```python
from build123d import *

# Parameters (mm, degrees)
SKETCH1_W           = 400
SKETCH1_H           = 76.2
BOSS_EXTRUDE1_DEPTH = 50.8
SKETCH3_R           = 6.75
CUT_EXTRUDE2_DEPTH  = 50.8
SKETCH5_R           = 16
CUT_EXTRUDE3_DEPTH  = 77.2


with BuildPart() as part:
    # Sketch1 → Boss-Extrude1 (new body)
    with BuildSketch(Plane(origin=(0, 0, 0), x_dir=(1, 0, 0), z_dir=(0, 1, 0))):
        with Locations((200, 38.1)):
            Rectangle(SKETCH1_W, SKETCH1_H)
    extrude(amount=BOSS_EXTRUDE1_DEPTH)

    # Sketch3 → Cut-Extrude2 (cut)
    with BuildSketch(Plane(origin=(0, 50.8, 0), x_dir=(1, 0, 0), z_dir=(0, 1, 0))):
        with Locations((25, 63)):
            Circle(SKETCH3_R)
        with Locations((25, 13)):
            Circle(SKETCH3_R)
        with Locations((375, 63)):
            Circle(SKETCH3_R)
        with Locations((375, 13)):
            Circle(SKETCH3_R)
    extrude(amount=-CUT_EXTRUDE2_DEPTH, mode=Mode.SUBTRACT)

    # Sketch5 → Cut-Extrude3 (cut, through all)
    with BuildSketch(Plane.XY):
        with Locations((200, 30)):
            Circle(SKETCH5_R)
        with Locations((70, 30)):
            Circle(SKETCH5_R)
        with Locations((330, 30)):
            Circle(SKETCH5_R)
    extrude(amount=-CUT_EXTRUDE3_DEPTH, mode=Mode.SUBTRACT)


solid = part.part
```
For this review, take the finished solid that the model builds, in its own axes (mm). Give positions to 0.01 mm unless a question says otherwise; leave off trailing zeros. Write each loop counter-clockwise with the first axis right and the second up, starting at its lowest first coordinate (ties: lowest second). Pieces come first, ordered by that corner, then holes.
Item 1: Take a section at A-A (x = 375). Give the boundary of the cut face in (y, z), and give its area (3 significant figures).
Item 2: Take a section at B-B (z = -63). Give the boundary of the cut face in (x, y).
Item 3: Wall thickness on probe 1 along Z at (x, y) = (374, 24); probe 2 along X at (y, z) = (29.5, -20); probe 3 along X at (y, z) = (9, -18): over which ranges is each line inside the solid? List them lowest first.
Item 4: The part is to be moulded in two halves that separate along X. For faces 1 (the face through (0, 25, -38)), 2 (the face through (197, 14, -76.2)), 3 (the face through (57.303, 20.264, -37.567)), say which applies: +X half, -X half, draft (parallel to the pull), parting line (faces both ways), or undercut.
Item 5: Insertion check: P1, Ø1.5, axis at x = 290, z = -44.5, coming from the -Y side; P2, Ø8, axis at x = 80, y = 28, coming from the +Z side. Each pin has a flat end and moves straight along its axis. Give the tip position at first contact, or say it passes through.
Item 6: Take a section at D-D (y = 37.5). Give the boundary of the cut face in (x, z).
Item 7: Take a section at C-C (y = 7.5). Give the boundary of the cut face in (x, z), and give its area (3 significant figures).
Established:
1. outline: (0, -76.2) - (50.8, -76.2) - (50.8, -69.75) - (0, -69.75) - close; (0, -56.25) - (50.8, -56.25) - (50.8, -19.75) - (0, -19.75) - close; (0, -6.25) - (50.8, -6.25) - (50.8, 0) - (0, 0) - close
1. area: 2,500 mm2
2. outline: (0, 0) - (18.25, 0) - (18.25, 50.8) - (0, 50.8) - close; (31.75, 0) - (368.25, 0) - (368.25, 50.8) - (31.75, 50.8) - close; (381.75, 0) - (400, 0) - (400, 50.8) - (381.75, 50.8) - close; hole circle Ø32 at (70, 30); hole circle Ø32 at (200, 30); hole circle Ø32 at (330, 30)
3. probe 1: z = -76.2 to -69.68, -56.32 to -19.68, -6.32 to 0
3. probe 2: x = 0 to 54.01, 85.99 to 184.01, 215.99 to 314.01, 345.99 to 400
3. probe 3: x = 0 to 20.47, 29.53 to 370.47, 379.53 to 400
4. face 1: -X half
4. face 2: draft
4. face 3: undercut
5. P1: stops at y = 0
5. P2: passes through
6. outline: (0, -76.2) - (55.87, -76.2) - (55.87, 0) - (0, 0) - close; (84.13, -76.2) - (185.87, -76.2) - (185.87, 0) - (84.13, 0) - close; (214.13, -76.2) - (315.87, -76.2) - (315.87, 0) - (214.13, 0) - close; (344.13, -76.2) - (400, -76.2) - (400, 0) - (344.13, 0) - close; hole circle Ø13.5 at (25, -63); hole circle Ø13.5 at (25, -13); hole circle Ø13.5 at (375, -63); hole circle Ø13.5 at (375, -13)
7. outline: (0, -76.2) - (400, -76.2) - (400, 0) - (0, 0) - close; hole circle Ø13.5 at (25, -63); hole circle Ø13.5 at (25, -13); hole circle Ø13.5 at (375, -63); hole circle Ø13.5 at (375, -13)
7. area: 29,900 mm2
